Autodesk Inventor part; units mm, degrees
ref_plane "YZ Plane" through (0, 0, 0) normal (1, 0, 0) x (0, 1, 0)
ref_plane "XZ Plane" through (0, 0, 0) normal (0, 1, 0) x (-1, 0, 0)
ref_plane "XY Plane" through (0, 0, 0) normal (0, 0, 1) x (1, 0, 0)
sketch "Sketch1" plane through (0, 0, 0) normal (1, 0, 0) x (0, 1, 0)
  line L0 (-12.5, -22) -> (12.5, -22)
  line L1 (12.5, -22) -> (12.5, 22)
  line L2 (12.5, 22) -> (-12.5, 22)
  line L3 (-12.5, 22) -> (-12.5, -22)
  line L4 (-12.5, -22) -> (12.5, 22) construction
  line L5 (12.5, -22) -> (-12.5, 22) construction
  point P0 (0, 0)
  dimension "d0" = 25
  dimension "d1" = 44
extrude "Extrusion1" add sketch "Sketch1" along normal blind 3
sketch "Sketch2" plane through (0, 0, 0) normal (-1, 0, 0) x (0, 0, 1)
  line L0 (-5, -12.5) -> (5, -12.5)
  line L1 (5, -12.5) -> (5, -15.5)
  line L2 (5, -15.5) -> (-5, -15.5)
  line L3 (-5, -15.5) -> (-5, -12.5)
  line L4 (22, -12.5) -> (-22, -12.5)
  point P0 (0, 0)
  point P1 (0, -15.5)
  dimension "d4" = 10
  dimension "d5" = 3
extrude "Extrusion2" add sketch "Sketch2" against normal blind 3
sketch "Sketch3" plane through (0, 0, 0) normal (-1, 0, 0) x (0, 0, 1)
  line L0 (22, 12.5) -> (22, -12.5)
  line L1 (22, 5) -> (19, 5)
  line L2 (19, 5) -> (19, -5)
  line L3 (19, -5) -> (22, -5)
  line L4 (22, -5) -> (22, 5)
  point P0 (0, 0)
  point P1 (19, 0)
  dimension "d8" = 3
  dimension "d9" = 10
extrude "Extrusion3" cut sketch "Sketch3" against normal blind 3
mirror "Mirror1" about plane through (0, 0, 0) normal (0, 0, 1) of "Extrusion3"
properties part number "battery holder ends"
Geometry: final body of the model. Coordinates: model frame, mm. A direction names the side the tool comes from. Give positions to 0.01 mm unless a question says otherwise; leave off trailing zeros. Write each loop counter-clockwise with the first axis right and the second up, starting at its lowest first coordinate (ties: lowest second). Pieces come first, ordered by that corner, then holes. Notation, with made-up numbers: (55.25, 52.5) -> (95.25, 52.5) arc R5 ccw to (95.25, 59.5) -> close; hole circle Ø4 at (-26.5, 55.25). An arc over 180 degrees is marked (long way). Answer as a JSON object with one key per item and string values.
1. Contact query for flat-ended pins moving along their axis: pin 1 (0.9 mm diameter, centred on x = 1.5, y = 0, fed in from +Z); pin 2 (1.5 mm diameter, centred on x = 2, z = -16.5, fed in from -Y); pin 3 (1 mm diameter, centred on x = 1, y = -2, fed in from -Z). Output: stop coordinate, or through.
Ans:
{"pin 1": "stops at z = 19", "pin 2": "stops at y = -12.5", "pin 3": "stops at z = -19"}
2. Cut plane D-D on z = -5.5. Output: boundary loops of the cut face in (x, y).
Ans:
{"outline": "(0, -12.5) -> (3, -12.5) -> (3, 12.5) -> (0, 12.5) -> close"}
3. Access query for faces 1 (the flat face through (1, -12.5, -13)), 2 (the flat face through (1, -14, 5)), 3 (the flat face through (1, 12.5, 0)), 4 (the flat face through (1, -5, 20)), 5 (the flat face through (1, 5, -20)). Directions: +Z, -Z, +X, -X, +Y, -Y. A direction counts if a zero-diameter tool reaches every point of the face in a straight line with its end or side. Return the directions, or none.
Ans:
{"face 1": "-Z, +X, -X, -Y", "face 2": "+Z, +X, -X, -Y", "face 3": "+Z, -Z, +X, -X, +Y", "face 4": "+Z, +X, -X", "face 5": "-Z, +X, -X"}
4. Cut plane C-C on y = -13.75. Output: boundary loops of the cut face in (x, z), and give its area (3 significant figures).
Ans:
{"outline": "(0, -5) -> (3, -5) -> (3, 5) -> (0, 5) -> close", "area": "30.0 mm^2"}
5. Cut plane B-B on x = 1.05. Output: boundary loops of the cut face in (y, z).
Ans:
{"outline": "(-15.5, -5) -> (-12.5, -5) -> (-12.5, -22) -> (-5, -22) -> (-5, -19) -> (5, -19) -> (5, -22) -> (12.5, -22) -> (12.5, 22) -> (5, 22) -> (5, 19) -> (-5, 19) -> (-5, 22) -> (-12.5, 22) -> (-12.5, 5) -> (-15.5, 5) -> close"}
6. Cut plane A-A on z = 19.5. Output: boundary loops of the cut face in (x, y).
Ans:
{"outline": "(0, -12.5) -> (3, -12.5) -> (3, -5) -> (0, -5) -> close; (0, 5) -> (3, 5) -> (3, 12.5) -> (0, 12.5) -> close"}
7. Ray query, probe 1 along Y at (x, z) = (1.3, 14.5); probe 2 along Z at (x, y) = (1.7, 3); probe 3 along Z at (x, y) = (1.6, -13). Return the intervals inside material, ascending. Write a range as from..to.
Ans:
{"probe 1": "y = -12.5..12.5", "probe 2": "z = -19..19", "probe 3": "z = -5..5"}
8. Mould query, pull axis Y, two halves, no side actions, for faces 6 (the flat face through (1, 0, -19)), 7 (the flat face through (1, -15.5, 0)), 8 (the flat face through (3, -2, 0)). Classes: pulls with the +Y half, pulls with the -Y half, needs draft (parallel to the pull), parting line crosses it, or undercut.
Ans:
{"face 6": "undercut", "face 7": "pulls with the -Y half", "face 8": "needs draft"}
